Here's how the part is built. I have some questions about the finished solid (model axes, mm). A direction names the side the tool comes from. Give positions to 0.01 mm unless a question says otherwise; leave off trailing zeros. Write each loop counter-clockwise with the first axis right and the second up, starting at its lowest first coordinate (ties: lowest second). Pieces come first, ordered by that corner, then holes. Notation, with made-up numbers: (28, 7.5) - (57, 7.5) arc R13 cw to (57, 18.5) - close; hole circle Ø2 at (11, 25). An arc over 180 degrees is marked (long way). Use one line per item in the form item = value. Start each with the question number.
from build123d import *

# Parameters (mm, degrees)
F1_DEPTH     = 63.5
F2_DEPTH     = 12.7
F2_FACE_W    = 69.919578209
F2_FACE_H    = 25.4
F4_T1_DEPTH  = 134.62
F4_T3_DEPTH  = 53.34
F4_T5_DEPTH  = 45.72
F4_T7_DEPTH  = 16.9064607487
F4_T9_DEPTH  = 63.5
F4_T11_DEPTH = 88.9
F4_T13_DEPTH = 109.22
F4_S17_W     = 5.08
F4_S17_H     = 5.08
F4_T18_DEPTH = 5.08
F4_S23_W     = 5.08
F4_S23_H     = 5.08
F4_T24_DEPTH = 5.08
F4_T28_ANGLE = 152.7793054157
F4_T30_ANGLE = 152.7793054157
F4_T35_DEPTH = 58.42
F4_T39_DEPTH = 29.6064607487
F4_T46_DEPTH = 76.2
F4_T50_DEPTH = 29.6064607487


# Not quite as in the source:
# - a fillet or chamfer that OpenCascade refuses, or shapes differently, is made with other operations: its cross-section is extruded or revolved along the edge and cut away or added


with BuildPart() as f1:
    # F0 (on Front) → F1 (new body, symmetric)
    with BuildSketch(Plane.XZ):
        Polygon((-50.8, 31.75), (-50.8, -31.75), (50.8, -31.75), (50.8, 31.75), (25.4, 31.75), align=None)
    extrude(amount=F1_DEPTH, both=True)

    # F0 (on Front) → F2 (join, symmetric)
    with BuildSketch(Plane.XZ):
        with BuildLine():
            add(Edge.make_bspline(
                [(-50.8, 31.75), (-12.3217052749, 49.9639766453), (18.113411963, 91.8597280979), (64.6348841752, 86.3919299359)],
                knots=[0, 0, 0, 0, 127.7143413704, 127.7143413704, 127.7143413704, 127.7143413704], degree=3))
            Line((-50.8, 31.75), (25.4, 31.75))
            Line((25.4, 31.75), (25.4, 48.6564607487))
            ThreePointArc((25.4, 48.6564607487), (36.9860122893, 75.8747531778), (64.6348841752, 86.3919299359))
        make_face()
        with BuildLine():
            Line((25.4, 31.75), (50.8, 31.75))
            Line((50.8, 31.75), (50.8, 48.6564607487))
            ThreePointArc((50.8, 48.6564607487), (54.7240260068, 57.691740436), (64.0053517954, 60.9919299359))
            Line((64.0053517954, 60.9919299359), (81.6413929723, 60.9919299359))
            Line((81.6413929723, 60.9919299359), (81.6413929723, 86.3919299359))
            Line((81.6413929723, 86.3919299359), (64.6348841752, 86.3919299359))
            ThreePointArc((64.6348841752, 86.3919299359), (36.9860122893, 75.8747531778), (25.4, 48.6564607487))
            Line((25.4, 48.6564607487), (25.4, 31.75))
        make_face()
        Polygon((81.6413929723, 98.0887729745), (81.6413929723, 86.3919299359), (81.6413929723, 60.9919299359), (81.6413929723, 49.5563661095), (151.5609711813, 49.5563661095), (151.5609711813, 98.0887729745), align=None)
    extrude(amount=F2_DEPTH, both=True)

    # F2_face (on face) → F3 (revolve)
    with BuildSketch(Plane(origin=(116.6011820768, 0, 98.0887729745), x_dir=(1, 0, 0), z_dir=(0, 0, 1))):
        Rectangle(F2_FACE_W, F2_FACE_H)
    revolve(axis=Axis((151.5609711813, 0, 98.0887729745), (0, -1, 0)))

    # F4: fillet of radius 5.08 on 13 edges, made by hand

    # F4_s2 → F4_t1 (cut)
    with BuildSketch(Plane.XZ.offset(-58.42)):
        with BuildLine():
            ThreePointArc((45.72, -31.75), (49.3121024484, -30.2621024484), (50.8, -26.67))
            Line((50.8, -26.67), (50.8, -31.75))
            Line((50.8, -31.75), (45.72, -31.75))
        make_face()
    extrude(amount=F4_T1_DEPTH, mode=Mode.SUBTRACT)

    # F4_s4 → F4_t3 (cut)
    with BuildSketch(Plane.XY.offset(-26.67)):
        with BuildLine():
            ThreePointArc((45.72, 63.5), (49.3121024484, 62.0121024484), (50.8, 58.42))
            Line((50.8, 58.42), (50.8, 63.5))
            Line((50.8, 63.5), (45.72, 63.5))
        make_face()
    extrude(amount=F4_T3_DEPTH, mode=Mode.SUBTRACT)

    # F4_s6 → F4_t5 (cut)
    with BuildSketch(Plane.XZ.offset(-58.42)):
        with BuildLine():
            ThreePointArc((45.72, 31.75), (49.3121024484, 30.2621024484), (50.8, 26.67))
            Line((50.8, 26.67), (50.8, 31.75))
            Line((50.8, 31.75), (45.72, 31.75))
        make_face()
    extrude(amount=F4_T5_DEPTH, mode=Mode.SUBTRACT)

    # F4_s8 → F4_t7 (cut)
    with BuildSketch(Plane.XY.offset(31.75)):
        with BuildLine():
            ThreePointArc((50.8, 7.62), (49.3121024484, 11.2121024484), (45.72, 12.7))
            Line((45.72, 12.7), (50.8, 12.7))
            Line((50.8, 12.7), (50.8, 7.62))
        make_face()
        with BuildLine():
            ThreePointArc((50.8, -7.62), (49.3121024484, -11.2121024484), (45.72, -12.7))
            Line((45.72, -12.7), (50.8, -12.7))
            Line((50.8, -12.7), (50.8, -7.62))
        make_face()
    extrude(amount=F4_T7_DEPTH, mode=Mode.SUBTRACT)

    # F4_s10 → F4_t9 (cut)
    with BuildSketch(Plane.XZ.offset(12.7)):
        with BuildLine():
            ThreePointArc((45.72, 31.75), (49.3121024484, 30.2621024484), (50.8, 26.67))
            Line((50.8, 26.67), (50.8, 31.75))
            Line((50.8, 31.75), (45.72, 31.75))
        make_face()
    extrude(amount=F4_T9_DEPTH, mode=Mode.SUBTRACT)

    # F4_s12 → F4_t11 (cut)
    with BuildSketch(Plane.XY.offset(-44.45)):
        with BuildLine():
            ThreePointArc((45.72, -63.5), (49.3121024484, -62.0121024484), (50.8, -58.42))
            Line((50.8, -58.42), (50.8, -63.5))
            Line((50.8, -63.5), (45.72, -63.5))
        make_face()
        with BuildLine():
            ThreePointArc((-50.8, 58.42), (-49.3121024484, 62.0121024484), (-45.72, 63.5))
            Line((-45.72, 63.5), (-50.8, 63.5))
            Line((-50.8, 63.5), (-50.8, 58.42))
        make_face()
    extrude(amount=F4_T11_DEPTH, mode=Mode.SUBTRACT)

    # F4_s14 → F4_t13 (cut)
    with BuildSketch(Plane.YZ.offset(-63.5)):
        with BuildLine():
            ThreePointArc((63.5, -26.67), (62.0121024484, -30.2621024484), (58.42, -31.75))
            Line((58.42, -31.75), (63.5, -31.75))
            Line((63.5, -31.75), (63.5, -26.67))
        make_face()
        with BuildLine():
            ThreePointArc((63.5, 26.67), (62.0121024484, 30.2621024484), (58.42, 31.75))
            Line((58.42, 31.75), (63.5, 31.75))
            Line((63.5, 31.75), (63.5, 26.67))
        make_face()
    extrude(amount=F4_T13_DEPTH, mode=Mode.SUBTRACT)


with BuildPart() as f4_tool16:
    # F4_s17 → F4_t18 (new body)
    with BuildSketch(Plane.YZ.offset(45.72)):
        with Locations((60.96, -29.21)):
            Rectangle(F4_S17_W, F4_S17_H)
    extrude(amount=F4_T18_DEPTH)

    # F4_s19 → F4_t20 (revolve, cut)
    with BuildSketch(Plane(origin=(45.72, 58.42, -26.67), x_dir=(0, -0.7071067812, 0.7071067812), z_dir=(0, 0.7071067812, 0.7071067812))):
        with BuildLine():
            ThreePointArc((0, -5.08), (5.08, 0), (0, 5.08))
            Line((0, 5.08), (0, -5.08))
        make_face()
    revolve(axis=Axis((45.72, 58.42, -26.67), (1, 0, 0)), mode=Mode.SUBTRACT)


with BuildPart() as f1_1:
    add(f1.part)

    # F4_t15: cut F4_tool16
    add(f4_tool16.part, mode=Mode.SUBTRACT)


with BuildPart() as f4_tool22:
    # F4_s23 → F4_t24 (new body)
    with BuildSketch(Plane.YZ.offset(45.72)):
        with Locations((60.96, 29.21)):
            Rectangle(F4_S23_W, F4_S23_H)
    extrude(amount=F4_T24_DEPTH)

    # F4_s25 → F4_t26 (revolve, cut)
    with BuildSketch(Plane(origin=(45.72, 58.42, 26.67), x_dir=(0, -0.7071067812, -0.7071067812), z_dir=(0, -0.7071067812, 0.7071067812))):
        with BuildLine():
            ThreePointArc((0, -5.08), (5.08, 0), (0, 5.08))
            Line((0, 5.08), (0, -5.08))
        make_face()
    revolve(axis=Axis((45.72, 58.42, 26.67), (1, 0, 0)), mode=Mode.SUBTRACT)


with BuildPart() as f1_2:
    add(f1_1.part)

    # F4_t21: cut F4_tool22
    add(f4_tool22.part, mode=Mode.SUBTRACT)

    # F4_s27 → F4_t28 (revolve, cut)
    with BuildSketch(Plane.XY.offset(48.6564607487)):
        with BuildLine():
            ThreePointArc((45.72, -12.7), (49.3121024484, -11.2121024484), (50.8, -7.62))
            Line((50.8, -7.62), (50.8, -12.7))
            Line((50.8, -12.7), (45.72, -12.7))
        make_face()
    revolve(axis=Axis((63.1641202888, -12.7, 48.6564607487), (0, 1, 0)), revolution_arc=F4_T28_ANGLE, mode=Mode.SUBTRACT)

    # F4_s29 → F4_t30 (revolve, cut)
    with BuildSketch(Plane.XY.offset(48.6564607487)):
        with BuildLine():
            ThreePointArc((45.72, 12.7), (49.3121024484, 11.2121024484), (50.8, 7.62))
            Line((50.8, 7.62), (50.8, 12.7))
            Line((50.8, 12.7), (45.72, 12.7))
        make_face()
    revolve(axis=Axis((63.1641202888, 12.7, 48.6564607487), (0, 1, 0)), revolution_arc=F4_T30_ANGLE, mode=Mode.SUBTRACT)


with BuildPart() as f4_tool33:
    # F4_s34 → F4_t35 (new body)
    with BuildSketch(Plane.XZ):
        with BuildLine():
            ThreePointArc((45.72, 31.75), (49.3121024484, 30.2621024484), (50.8, 26.67))
            Line((50.8, 26.67), (50.8, 31.75))
            Line((50.8, 31.75), (45.72, 31.75))
        make_face()
    extrude(amount=-F4_T35_DEPTH)

    split(bisect_by=Plane.XZ.offset(-12.7), keep=Keep.TOP)


with BuildPart() as f4_tool37:
    # F4_s38 → F4_t39 (new body)
    with BuildSketch(Plane.XY.offset(19.05)):
        with BuildLine():
            ThreePointArc((50.8, 7.62), (49.3121024484, 11.2121024484), (45.72, 12.7))
            Line((45.72, 12.7), (50.8, 12.7))
            Line((50.8, 12.7), (50.8, 7.62))
        make_face()
    extrude(amount=F4_T39_DEPTH)

    split(bisect_by=Plane.XY.offset(31.75), keep=Keep.BOTTOM)


with BuildPart() as f4_tool33_1:
    add(f4_tool33.part)

    # F4_t41: intersect F4_tool37
    add(f4_tool37.part, mode=Mode.INTERSECT)


with BuildPart() as f1_3:
    add(f1_2.part)

    # F4_t31: cut F4_tool33
    add(f4_tool33_1.part, mode=Mode.SUBTRACT)


with BuildPart() as f4_tool44:
    # F4_s45 → F4_t46 (new body)
    with BuildSketch(Plane.XZ.offset(76.2)):
        with BuildLine():
            ThreePointArc((45.72, 31.75), (49.3121024484, 30.2621024484), (50.8, 26.67))
            Line((50.8, 26.67), (50.8, 31.75))
            Line((50.8, 31.75), (45.72, 31.75))
        make_face()
    extrude(amount=-F4_T46_DEPTH)

    split(bisect_by=Plane.XZ.offset(12.7), keep=Keep.BOTTOM)


with BuildPart() as f4_tool48:
    # F4_s49 → F4_t50 (new body)
    with BuildSketch(Plane.XY.offset(19.05)):
        with BuildLine():
            ThreePointArc((50.8, -7.62), (49.3121024484, -11.2121024484), (45.72, -12.7))
            Line((45.72, -12.7), (50.8, -12.7))
            Line((50.8, -12.7), (50.8, -7.62))
        make_face()
    extrude(amount=F4_T50_DEPTH)

    split(bisect_by=Plane.XY.offset(31.75), keep=Keep.BOTTOM)


with BuildPart() as f4_tool44_1:
    add(f4_tool44.part)

    # F4_t52: intersect F4_tool48
    add(f4_tool48.part, mode=Mode.INTERSECT)


with BuildPart() as f1_4:
    add(f1_3.part)

    # F4_t42: cut F4_tool44
    add(f4_tool44_1.part, mode=Mode.SUBTRACT)


solid = f1_4.part
1. For P1, Ø3, axis at x = 193, z = 53.5, coming from the -Y side; P2, Ø21.5, axis at x = 91, y = -4, coming from the -Z side; P3, Ø3.5, axis at y = -1.5, z = 56, coming from the -X side; P4, Ø10, axis at x = 130, y = 20.5, coming from the +Z side, each with a flat end and sliding along its axis, tell me the tip position at first contact or that it passes through.
2. I want a section at C-C, the plane x = 112.5. List the corners of the cut face in (y, z) for me.
3. I want a section at A-A, the plane z = 8.5. List the corners of the cut face in (x, y) for me.
4. We'd pull the mould along X, two halves only. Please class faces 1 (the face through (-3, -3, -31.75)), 2 (the face through (-50.8, -3, 0)), 3 (the face through (54.621, -0.107, 57.594)): pulls with the +X half, pulls with the -X half, needs draft (parallel to the pull), parting line crosses it, or undercut.
5. I want a section at B-B, the plane y = 50.5. List the corners of the cut face in (x, z) for me.
6. For faces 4 (the face through (73, 0, 86.392)), 5 (the face through (-2, 35, 31.75)), 6 (the face through (91, 0, 49.556)), 7 (the face through (-2, -38, 31.75)), 8 (the face through (-3, -63.5, 0)), which set-ups out of +Z, -Z, +X, -X, +Y, -Y let a thin tool reach every point of the face, with its end or its side?
7. I want a section at D-D, the plane z = 110. List the corners of the cut face in (x, y) for me, then the cut area to 3 significant figures.
8. Please list where these lines run through material, in increasing order: line 1 (X direction, y = -31, z = -15.5); line 2 (Y direction, x = 190, z = 98); line 3 (Z direction, x = 33, y = 14.5).
Result sheet:
q1.P1 = -12.7
q1.P2 = 49.02
q1.P3 = -15.45
q1.P4 = through
q2.outline = (-12.7, 40.1) - (12.7, 40.1) - (12.7, 156.08) - (-12.7, 156.08) - close
q3.outline = (-50.8, -63.5) - (45.72, -63.5) arc R5.08 ccw to (50.8, -58.42) - (50.8, 58.42) arc R5.08 ccw to (45.72, 63.5) - (-45.72, 63.5) arc R5.08 ccw to (-50.8, 58.42) - close
q4.face_1 = needs draft
q4.face_2 = pulls with the -X half
q4.face_3 = undercut
q5.outline = (-50.8, -31.75) - (45.72, -31.75) arc R5.08 ccw to (50.8, -26.67) - (50.8, 26.67) arc R5.08 ccw to (45.72, 31.75) - (-50.8, 31.75) - close
q6.face_4 = +Z, +Y, -Y
q6.face_5 = +Z, +X, -X, +Y
q6.face_6 = -Z, +Y, -Y
q6.face_7 = +Z, +X, -X, -Y
q6.face_8 = +Z, -Z, +X, -X, -Y
q7.outline = (82.66, -12.7) - (220.46, -12.7) - (220.46, 12.7) - (82.66, 12.7) - close
q7.area = 3,500 mm2
q8.line_1 = -50.8 to 50.8
q8.line_2 = -12.7 to 12.7
q8.line_3 = -31.75 to 31.75
